Geometry check sheet. Reference: the model listing, model coordinates, mm. Face numbers are marked on the shaded views. A direction names the side the tool comes from. Round coordinates to 2 decimals unless told otherwise and drop trailing zeros. Order: outer loops, then holes, each group sorted by start corner. A loop starts at its lowest first (then second) coordinate and runs counter-clockwise, first axis right, second up.
(1) Sectioned sample at B-B (x = 9.5). Record the boundary of the cut face in (y, z) (3 decimals), plus the area to 3 significant figures.
(2) Go/stop test with flat-tipped pins: pin 1 (1.9 mm diameter, centred on y = 13, z = 7.5, fed in from -X) (3 decimals); pin 2 (1.4 mm diameter, centred on y = 23, z = 9, fed in from -X); pin 3 (4.5 mm diameter, centred on x = 22, y = 39, fed in from -Z). Record where each tip stops, or that it passes through.
(3) Sectioned sample at C-C (y = 17.5). Record the boundary of the cut face in (x, z) (3 decimals), plus the area to 3 significant figures.
(4) Sectioned sample at D-D (y = 36). Record the boundary of the cut face in (x, z) (3 decimals).
(5) Release check for a two-part mould opening along X. For the marked faces 4, 5 and 6 record: +X half, -X half, draft (parallel to the pull), parting line (faces both ways), or undercut.
(6) Set-up check for the marked faces 1, 2 and 3: record each of +Z, -Z, +X, -X, +Y, -Y from which the full face is reachable in a straight line by a thin tool's end or side.
(7) Material ranges on line 1 along X through (y, z) = (7.5, 2.5); line 2 along X through (y, z) = (17, 7.25) (3 decimals); line 3 along X through (y, z) = (8.5, 5.25) (3 decimals), recorded low to high.
(8) Sectioned sample at A-A (z = 1.75). Record the boundary of the cut face in (x, y).
from build123d import *

# Parameters (mm, degrees)
F1_DEPTH = 3.048
F2_DEPTH = 8.2296
F0_R     = 2.3876
F3_DEPTH = 9.525
F4_R     = 4.699
F4_R_2   = 2.3876
F5_DEPTH = 6.5532


with BuildPart() as f1:
    # F0 (on Top) → F1 (new body)
    with BuildSketch(Plane.XY):
        Polygon((0, 44.196), (0, 0), (8.255, 0), (8.255, 9.144), (8.255, 37.973), (8.255, 44.196), align=None)
    extrude(amount=F1_DEPTH)

    # F0 (on Top) → F2 (join)
    with BuildSketch(Plane.XY):
        with BuildLine():
            Line((8.255, 37.973), (8.255, 9.144))
            Line((8.255, 9.144), (14.732, 9.144))
            ThreePointArc((14.732, 9.144), (19.311931, 11.041069), (21.209, 15.621))
            Line((21.209, 15.621), (21.209, 31.496))
            ThreePointArc((21.209, 31.496), (19.311931, 36.075931), (14.732, 37.973))
            Line((14.732, 37.973), (8.255, 37.973))
        make_face()
    extrude(amount=F2_DEPTH)

    # F0 (on Top) → F3 (join)
    with BuildSketch(Plane.XY):
        with BuildLine():
            Line((8.255, 9.144), (8.255, 0))
            Line((8.255, 0), (97.536, 0))
            Line((97.536, 0), (97.536, 44.196))
            Line((97.536, 44.196), (8.255, 44.196))
            Line((8.255, 44.196), (8.255, 37.973))
            Line((8.255, 37.973), (14.732, 37.973))
            ThreePointArc((14.732, 37.973), (19.311931, 36.075931), (21.209, 31.496))
            Line((21.209, 31.496), (21.209, 15.621))
            ThreePointArc((21.209, 15.621), (19.311931, 11.041069), (14.732, 9.144))
            Line((14.732, 9.144), (8.255, 9.144))
        make_face()
        with Locations((19.6596, 5.6896)):
            Circle(F0_R, mode=Mode.SUBTRACT)
        with Locations((69.7484, 6.146022)):
            Circle(F0_R, mode=Mode.SUBTRACT)
        with Locations((22.3266, 39.7764)):
            Circle(F0_R, mode=Mode.SUBTRACT)
        with Locations((66.8274, 39.7764)):
            Circle(F0_R, mode=Mode.SUBTRACT)
    extrude(amount=F3_DEPTH)

    # F4 (on face) → F5 (cut)
    with BuildSketch(Plane.XY):
        with Locations((69.7484, 6.146022)):
            Circle(F4_R)
        with Locations((19.6596, 5.6896)):
            Circle(F4_R)
        with BuildLine():
            Line((71.525994, 39.838142), (71.525994, 44.196))
            Line((71.525994, 44.196), (62.128806, 44.196))
            Line((62.128806, 44.196), (62.128806, 39.838142))
            ThreePointArc((62.128806, 39.838142), (66.8274, 35.0774), (71.525994, 39.838142))
        make_face()
        with Locations((66.8274, 39.7764)):
            Circle(F4_R_2, mode=Mode.SUBTRACT)
        with BuildLine():
            Line((27.016125, 44.196), (17.637075, 44.196))
            Line((17.637075, 44.196), (17.637075, 39.478143))
            ThreePointArc((17.637075, 39.478143), (22.3266, 35.0774), (27.016125, 39.478143))
            Line((27.016125, 39.478143), (27.016125, 44.196))
        make_face()
        with Locations((22.3266, 39.7764)):
            Circle(F4_R_2, mode=Mode.SUBTRACT)
    extrude(amount=F5_DEPTH, mode=Mode.SUBTRACT)


solid = f1.part
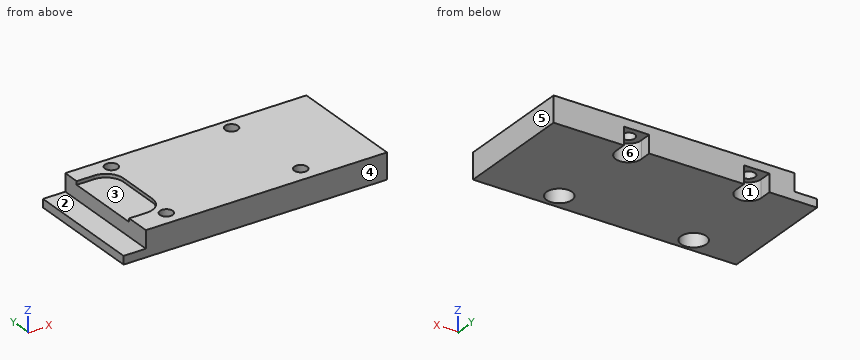
Answer below:
1. outline: (0, 0) - (44.196, 0) - (44.196, 9.525) - (37.973, 9.525) - (37.973, 8.23) - (9.144, 8.23) - (9.144, 9.525) - (0, 9.525) - close
1. area: 384 mm2
2. pin 1: stops at x = 8.255
2. pin 2: stops at x = 21.21
2. pin 3: stops at z = 6.55
3. outline: (0, 0) - (97.536, 0) - (97.536, 9.525) - (21.209, 9.525) - (21.209, 8.23) - (8.255, 8.23) - (8.255, 3.048) - (0, 3.048) - close
3. area: 859 mm2
4. outline: (0, 0) - (19.53, 0) - (19.53, 6.553) - (25.123, 6.553) - (25.123, 0) - (64.031, 0) - (64.031, 6.553) - (69.624, 6.553) - (69.624, 0) - (97.536, 0) - (97.536, 9.525) - (19.387, 9.525) - (19.387, 8.23) - (8.255, 8.23) - (8.255, 3.048) - (0, 3.048) - close
5. face 4: draft
5. face 5: +X half
5. face 6: undercut
6. face 1: -Z, +Y
6. face 2: +Z, -X, +Y, -Y
6. face 3: +Z, -X
7. line 1: x = 0 to 15.32, 24 to 65.25, 74.25 to 97.54
7. line 2: x = 8.255 to 97.536
7. line 3: x = 8.255 to 15.894, 23.426 to 65.682, 73.815 to 97.536
8. outline: (0, 0) - (97.54, 0) - (97.54, 44.2) - (71.53, 44.2) - (71.53, 39.84) arc R4.7 cw (long way) to (62.13, 39.84) - (62.13, 44.2) - (27.02, 44.2) - (27.02, 39.48) arc R4.7 cw to (17.64, 39.48) - (17.64, 44.2) - (0, 44.2) - close; hole circle Ø9.4 at (19.66, 5.69); hole circle Ø9.4 at (69.75, 6.15)
